Can you work these out from the model? Positions are in its coordinate system, mm. Face numbers are marked on the shaded views. Coordinates: 2 decimals unless noted, no trailing zeros. Order: outer loops, then holes, each group sorted by start corner. A loop starts at its lowest first (then second) coordinate and runs counter-clockwise, first axis right, second up. Notation, with made-up numbers: (-28, 57.25) -> (-5, 57.25) arc R12 cw to (-5, 79.25) -> close; hole circle Ø6 at (67, -35). An arc over 180 degrees is marked (long way). Return JSON: item names as keys, results as strings. Group by question number.
1) If I drill on probe 1 along Y at (x, z) = (-99.75, 11); probe 2 along Y at (x, z) = (-100, 7.5); probe 3 along X at (y, z) = (-19.5, 28.5), over which ranges is the centre line in solid material (lowest first)? Write a range as from..to.
2) If we section it at A-A, the plane x = -95: Please give me the cut outline in (y, z).
3) If we section it at B-B, the plane x = -99.25: Please give me the cut outline in (y, z), then the cut area to 3 significant figures.
4) Thinking about a two-plate mould opening in Z: for the marked faces 1, 2 and 3, which applies, +Z half, -Z half, draft (parallel to the pull), parting line (faces both ways), or undercut?
5) For pin 1 (6 mm diameter, centred on y = -15, z = 8, fed in from +X); pin 2 (1 mm diameter, centred on x = -92.5, z = -13, fed in from +Y); pin 3 (2 mm diameter, centred on x = -87, y = -41.5, fed in from -Z), each with a flat end and sliding along its axis, tell me the tip position at first contact or that it passes through.
6) If we section it at C-C, the plane x = -103.25: Please give me the cut outline in (y, z), then the cut area to 3 significant figures.
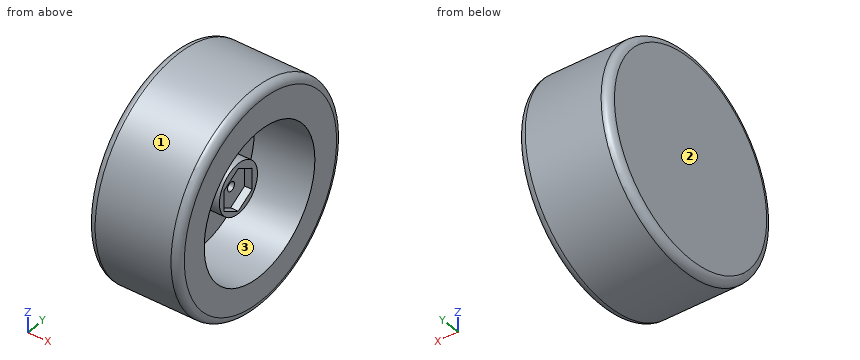
from build123d import *

# Parameters (mm, degrees)
SKETCH034_R     = 35.5
PAD014_DEPTH    = 30
FILLET018_R     = 2.5
FILLET019_R     = 2.5
SKETCH035_R     = 24
POCKET003_DEPTH = 20
SKETCH036_R     = 8.25
PAD015_DEPTH    = 12
POCKET004_DEPTH = 2.5
SKETCH038_R     = 1.5
POCKET005_DEPTH = 3.5


with BuildPart() as part:
    # Sketch034 → Pad014 (new body)
    with BuildSketch(Plane.YZ):
        with Locations((-2.086276, 2.086154)):
            Circle(SKETCH034_R)
    extrude(amount=PAD014_DEPTH)

    # Fillet018
    fillet018_edges = [part.edges().sort_by_distance(p)[0] for p in [
        (30, -37.586276, 2.086154),
    ]]
    fillet(fillet018_edges, radius=FILLET018_R)

    # Fillet019
    fillet019_edges = [part.edges().sort_by_distance(p)[0] for p in [
        (0, -37.586276, 2.086154),
    ]]
    fillet(fillet019_edges, radius=FILLET019_R)

    # Sketch035 (on Face3 of Pad014) → Pocket003 (cut)
    with BuildSketch(Plane.YZ.offset(30)):
        with Locations((-2.490074, 1.413427)):
            Circle(SKETCH035_R)
    extrude(amount=-POCKET003_DEPTH, mode=Mode.SUBTRACT)

    # Sketch036 (on Face7 of Pocket003) → Pad015 (join)
    with BuildSketch(Plane.YZ.offset(10)):
        with Locations((-1.106776, 1.902246)):
            Circle(SKETCH036_R)
    extrude(amount=PAD015_DEPTH)

    # Sketch037 (on Face9 of Pad015) → Pocket004 (cut)
    with BuildSketch(Plane.YZ.offset(22)):
        Polygon((4.852949, 4.988847), (-1.209229, 8.488847), (-7.271407, 4.988847), (-7.271407, -2.011153), (-1.209229, -5.511153), (4.852949, -2.011153), align=None)
    extrude(amount=-POCKET004_DEPTH, mode=Mode.SUBTRACT)

    # Sketch038 (on Face16 of Pocket004) → Pocket005 (cut)
    with BuildSketch(Plane.YZ.offset(19.5)):
        with Locations((-1.040093, 1.343548)):
            Circle(SKETCH038_R)
    extrude(amount=-POCKET005_DEPTH, mode=Mode.SUBTRACT)


with BuildPart() as part_1:
    # Body002 placement: moved
    add(part.part.moved(Location((-112, -11, 5))))


solid = part_1.part
Result sheet:
{
 "1": {"probe 1": "y = -48.37..-37.05, -19.27..-4.95, 10.07..22.2", "probe 2": "y = -48.58..-37.47, -20.34..-3.88, 10.49..22.41", "probe 3": "x = -112..-102"},
 "2": {"outline": "circle Ø71 at (-13.09, 7.09); circle Ø16.5 at (-12.11, 6.9); hole circle Ø48 at (-13.49, 6.41); hole circle Ø3 at (-12.04, 6.34)"},
 "3": {"outline": "circle Ø71 at (-13.09, 7.09); circle Ø16.5 at (-12.11, 6.9); hole circle Ø48 at (-13.49, 6.41)", "area": "2,360 mm2"},
 "4": {"face 1": "parting line", "face 2": "draft", "face 3": "undercut"},
 "5": {"pin 1": "stops at x = -92.5", "pin 2": "stops at y = 16.52", "pin 3": "stops at z = -15.47"},
 "6": {"outline": "circle Ø71 at (-13.09, 7.09)", "area": "3,960 mm2"}
}
